from build123d import *

# Parameters (mm, degrees)
F0_W     = 12.5
F0_H     = 12
F1_DEPTH = 15
F2_W     = 8.215
F2_H     = 15
F3_DEPTH = 10
F4_W     = 5.3
F4_H     = 15
F5_DEPTH = 6.05


with BuildPart() as f1:
    # F0 (on Top) → F1 (new body)
    with BuildSketch(Plane.XY):
        with Locations((-6.25, 6)):
            Rectangle(F0_W, F0_H)
        Polygon((0, 12), (0, 0), (3.6608153082, -1.3324278053), (7.5175409663, 9.2638388534), align=None)
    extrude(amount=F1_DEPTH)

    # F2 (on face) → F3 (cut)
    with BuildSketch(Plane(origin=(-12.5, 0, 0), x_dir=(0, -1, 0), z_dir=(-1, 0, 0))):
        with Locations((-6, 7.5)):
            Rectangle(F2_W, F2_H)
    extrude(amount=-F3_DEPTH, mode=Mode.SUBTRACT)

    # F4 (on face) → F5 (cut)
    with BuildSketch(Plane(origin=(3.6608153082, -1.3324278053, 0), x_dir=(0.3420201433, 0.9396926208, 0), z_dir=(0.9396926208, -0.3420201433, 0))):
        with Locations((5.6381557247, 7.5)):
            Rectangle(F4_W, F4_H)
    extrude(amount=-F5_DEPTH, mode=Mode.SUBTRACT)


solid = f1.part
Input: part model. Units: mm. Frame: model coordinates. A direction names the side the tool comes from. Give positions to 0.01 mm unless a question says otherwise; leave off trailing zeros. Write each loop counter-clockwise with the first axis right and the second up, starting at its lowest first coordinate (ties: lowest second). Pieces come first, ordered by that corner, then holes. Notation, with made-up numbers: M 8.5,-34.5 L 21.5,-34.5 A20 cw 21.5,1.5 Z; hole C 4.5,84.25 d8. An arc over 180 degrees is marked long. Write item = value, one per line. Start each with the question number.
1) Reachability of faces 1 (the flat face through (1.88, 2.496, 7.395)), 2 (the flat face through (-2, 6, 0)), 3 (the flat face through (-8, 10.108, 7)), 4 (the flat face through (-0.11, 6, 7.6)), 5 (the flat face through (-6, 0, 7)) from +Z, -Z, +X, -X, +Y, -Y: full face, straight path, thin tool, end or side. Return the list, or none.
2) Cut plane A-A on x = -7.5. Return the cut outline in (y, z), then the cut area to 3 significant figures.
3) First-contact query: pin 1 Ø3 at (x, z) = (-8.5, 2.5) entering from -Y; pin 2 Ø8 at (x, z) = (2.5, 10.5) entering from -Y; pin 3 Ø5 at (y, z) = (5, 11.5) entering from +X. Flat tips, straight axial feed; report the tip coordinate or a pass-through.
4) Cut plane D-D on y = 9.75. Return the cut outline in (x, z), then the cut area to 3 significant figures.
5) Cut plane C-C on z = 13. Return the cut outline in (x, y).
6) Cut plane B-B on y = 7. Return the cut outline in (x, z), then the cut area to 3 significant figures.
7) Material intervals for line 1 along Y through (x, z) = (-5.5, 12); line 2 along Y through (x, z) = (1.5, 6.75); line 3 along Y through (x, z) = (-2, 2), sorted ascending. Write a range as [from, to].
Solved:
q1.face_1 = +Z, -Z, +X
q1.face_2 = -Z, +X, -X, +Y, -Y
q1.face_3 = +Z, -Z, -X
q1.face_4 = +Z, -Z
q1.face_5 = +Z, -Z, -X, -Y
q2.outline = M 0,0 L 1.89,0 L 1.89,15 L 0,15 Z; M 10.11,0 L 12,0 L 12,15 L 10.11,15 Z
q2.area = 56.8 mm2
q3.pin_1 = 0
q3.pin_2 = -1.33
q3.pin_3 = 6.88
q4.outline = M -2.5,0 L 6.18,0 L 6.18,15 L -2.5,15 Z
q4.area = 130 mm2
q5.outline = M -12.5,0 L 0,0 L 3.66,-1.33 L 4.68,1.48 L -1,3.54 L 0.81,8.53 L 6.5,6.46 L 7.52,9.26 L 0,12 L -12.5,12 L -12.5,10.11 L -2.5,10.11 L -2.5,1.89 L -12.5,1.89 Z
q6.outline = M -2.5,0 L 0.26,0 L 0.26,15 L -2.5,15 Z; M 5,0 L 6.69,0 L 6.69,15 L 5,15 Z
q6.area = 66.7 mm2
q7.line_1 = [0, 1.89], [10.11, 12]
q7.line_2 = [-0.55, 2.63], [8.27, 11.45]
q7.line_3 = [0, 12]
